from build123d import *

# Parameters (mm, degrees)
SKETCH1_W           = 40.5
SKETCH1_H           = 22
BOSS_EXTRUDE1_DEPTH = 3
SKETCH2_R           = 1
CUT_EXTRUDE1_DEPTH  = 10
SKETCH3_R           = 4
CUT_EXTRUDE2_DEPTH  = 10
SKETCH4_R           = 1
CUT_EXTRUDE3_DEPTH  = 10
SKETCH5_R           = 2
CUT_EXTRUDE4_DEPTH  = 1.5


with BuildPart() as part:
    # Sketch1 → Boss-Extrude1 (new body)
    with BuildSketch(Plane(origin=(0, 0, 0), x_dir=(1, 0, 0), z_dir=(0, 1, 0))):
        Rectangle(SKETCH1_W, SKETCH1_H)
    extrude(amount=BOSS_EXTRUDE1_DEPTH)

    # Sketch2 → Cut-Extrude1 (cut)
    with BuildSketch(Plane(origin=(0, 3, 0), x_dir=(1, 0, 0), z_dir=(0, 1, 0))):
        with Locations((-14.25, 8)):
            Circle(SKETCH2_R)
        with Locations((-14.25, -8)):
            Circle(SKETCH2_R)
        with Locations((14.25, -8)):
            Circle(SKETCH2_R)
        with Locations((14.25, 8)):
            Circle(SKETCH2_R)
    extrude(amount=-CUT_EXTRUDE1_DEPTH, mode=Mode.SUBTRACT)

    # Sketch3 → Cut-Extrude2 (cut)
    with BuildSketch(Plane(origin=(0, 3, 0), x_dir=(1, 0, 0), z_dir=(0, 1, 0))):
        Circle(SKETCH3_R)
    extrude(amount=-CUT_EXTRUDE2_DEPTH, mode=Mode.SUBTRACT)

    # Sketch4 → Cut-Extrude3 (cut)
    with BuildSketch(Plane(origin=(0, 3, 0), x_dir=(1, 0, 0), z_dir=(0, 1, 0))):
        with Locations((0, 7)):
            Circle(SKETCH4_R)
        with Locations((7, 0)):
            Circle(SKETCH4_R)
        with Locations((0, -7)):
            Circle(SKETCH4_R)
        with Locations((-7, 0)):
            Circle(SKETCH4_R)
    extrude(amount=-CUT_EXTRUDE3_DEPTH, mode=Mode.SUBTRACT)

    # Sketch5 → Cut-Extrude4 (cut)
    with BuildSketch(Plane(origin=(0, 3, 0), x_dir=(1, 0, 0), z_dir=(0, 1, 0))):
        with Locations((14.25, 8)):
            Circle(SKETCH5_R)
        with Locations((0, 7)):
            Circle(SKETCH5_R)
        with Locations((-14.25, 8)):
            Circle(SKETCH5_R)
        with Locations((7, 0)):
            Circle(SKETCH5_R)
        with Locations((-7, 0)):
            Circle(SKETCH5_R)
        with Locations((-14.25, -8)):
            Circle(SKETCH5_R)
        with Locations((0, -7)):
            Circle(SKETCH5_R)
        with Locations((14.25, -8)):
            Circle(SKETCH5_R)
    extrude(amount=-CUT_EXTRUDE4_DEPTH, mode=Mode.SUBTRACT)


solid = part.part
Read the model definition and answer for the solid it produces. Units are mm, in the model's axes. A direction names the side the tool comes from. Round coordinates to 2 decimals unless told otherwise and drop trailing zeros. Write each loop counter-clockwise with the first axis right and the second up, starting at its lowest first coordinate (ties: lowest second). Pieces come first, ordered by that corner, then holes. Notation, with made-up numbers: (87.5, 0) - (116.5, 0) arc R24 ccw to (116.5, 37) - close; hole circle Ø6 at (43, -23.75). An arc over 180 degrees is marked (long way). One line per question, with ' | ' between items. Start each with the question number.
1. For faces 1 (the face through (-6, 1.5, 1)), 2 (the face through (15.204, 0.76, -8.3)), determine the directions among +Z, -Z, +X, -X, +Y, -Y from which every point of the face is accessible in a straight line to the end or side of a thin tool.
2. Find the intervals of material crossed by probe 1 along X at (y, z) = (1.15, 0); probe 2 along Z at (x, y) = (14.25, 2.6); probe 3 along Z at (x, y) = (0, 1.65), in increasing order. Write a range as [from, to].
3. For a pull along Z with two mould halves and no side action, classify faces 3 (the face through (20.25, 1, 0)), 4 (the face through (-0.867, 1.521, 3.905)) as +Z half, -Z half, draft (parallel to the pull), parting line (faces both ways), or undercut.
4. Each of these flat-tipped pins is pushed along its axis until it touches: pin 1 (2.5 mm diameter, centred on x = 0, z = 7, fed in from -Y); pin 2 (1.2 mm diameter, centred on x = 14.5, z = -9, fed in from +Y). Where does it stop, or does it pass through?
5. Section C-C (z = 7.5) is taken. Determine the outline of the cut face in (x, y).
6. Section A-A (x = -7) is taken. Determine the outline of the cut face in (y, z), and give its area (3 significant figures).
7. Section D-D (x = 14.25) is taken. Determine the outline of the cut face in (y, z), and give its area (3 significant figures).
8. Section B-B (y = 0.85) is taken. Give the number of separate pieces and of enclosed holes in the cut face, and give its area (3 significant figures).
Filled in:
1) face 1: +Y | face 2: +Y, -Y
2) probe 1: [-20.25, -8], [-6, -4], [4, 6], [8, 20.25] | probe 2: [-11, -10], [-6, 6], [10, 11] | probe 3: [-11, -9], [-5, -4], [4, 5], [9, 11]
3) face 3: draft | face 4: undercut
4) pin 1: y = 0 | pin 2: y = 1.5
5) outline: (-20.25, 0) - (-15.12, 0) - (-15.12, 1.5) - (-16.19, 1.5) - (-16.19, 3) - (-20.25, 3) - close; (-13.38, 0) - (-0.87, 0) - (-0.87, 1.5) - (-1.94, 1.5) - (-1.94, 3) - (-12.31, 3) - (-12.31, 1.5) - (-13.38, 1.5) - close; (0.87, 0) - (13.38, 0) - (13.38, 1.5) - (12.31, 1.5) - (12.31, 3) - (1.94, 3) - (1.94, 1.5) - (0.87, 1.5) - close; (15.12, 0) - (20.25, 0) - (20.25, 3) - (16.19, 3) - (16.19, 1.5) - (15.12, 1.5) - close
6) outline: (0, -11) - (3, -11) - (3, -2) - (1.5, -2) - (1.5, -1) - (0, -1) - close; (0, 1) - (1.5, 1) - (1.5, 2) - (3, 2) - (3, 11) - (0, 11) - close | area: 57.0 mm²
7) outline: (0, -11) - (3, -11) - (3, -10) - (1.5, -10) - (1.5, -9) - (0, -9) - close; (0, -7) - (1.5, -7) - (1.5, -6) - (3, -6) - (3, 6) - (1.5, 6) - (1.5, 7) - (0, 7) - close; (0, 9) - (1.5, 9) - (1.5, 10) - (3, 10) - (3, 11) - (0, 11) - close | area: 48.0 mm²
8) separate pieces: 1 | enclosed holes: 9 | area: 816 mm²
